Check sheet for the modelled part. Datum: model origin and axes. Units: mm. A direction names the side the tool comes from. Give positions to 0.01 mm unless a question says otherwise; leave off trailing zeros. Loops run counter-clockwise (first coordinate to the right, second up) from the corner with the lowest first, then second, coordinate; pieces in that order, holes last.
Autodesk Inventor part; units mm, degrees
ref_plane "YZ Plane" through (0, 0, 0) normal (1, 0, 0) x (0, 1, 0)
ref_plane "XZ Plane" through (0, 0, 0) normal (0, 1, 0) x (-1, 0, 0)
ref_plane "XY Plane" through (0, 0, 0) normal (0, 0, 1) x (1, 0, 0)
sketch "Sketch1" plane through (0, 0, 0) normal (0, 0, 1) x (1, 0, 0)
  line L0 (0, 0) -> (43.18, 0)
  line L1 (43.18, 0) -> (43.18, 22.86)
  line L2 (43.18, 22.86) -> (0, 22.86)
  line L3 (0, 22.86) -> (0, 0)
  dimension "d0" = 43.18
  dimension "d1" = 22.86
extrude "Extrusion1" add sketch "Sketch1" along normal blind 24.892
sketch "Sketch2" plane through (43.18, 0, 0) normal (1, 0, 0) x (0, 0, -1)
  line L0 (-4.826, 5.08) -> (-14.986, 5.08)
  line L1 (-14.986, 5.08) -> (-14.986, 17.78)
  line L2 (-14.986, 17.78) -> (-4.826, 17.78)
  line L3 (-4.826, 17.78) -> (-4.826, 5.08)
  line L4 (-24.892, 0) -> (-24.892, 22.86) construction
  line L5 (-14.986, 8.255) -> (-20.066, 8.255)
  line L6 (-20.066, 8.255) -> (-20.066, 14.605)
  line L7 (-20.066, 14.605) -> (-14.986, 14.605)
  line L8 (-14.986, 14.605) -> (-14.986, 8.255)
  line L9 (-20.066, 17.78) -> (-4.826, 17.78)
  line L10 (0, 22.86) -> (-24.892, 22.86) construction
  point P0 (0, 0)
  point P1 (-14.986, 11.43)
  point P2 (-24.892, 11.43)
  point P3 (-20.066, 11.43)
  point P4 (-12.446, 17.78)
  point P5 (-12.446, 22.86)
  dimension "d4" = 10.16
  dimension "d5" = 12.7
  dimension "d6" = 5.08
  dimension "d7" = 6.35
extrude "Extrusion2" cut sketch "Sketch2" against normal blind 12.7
sketch "Sketch3" plane through (0, 0, 0) normal (-1, 0, 0) x (0, 0, 1)
  line L0 (14.986, 14.605) -> (14.986, 17.78)
  line L1 (20.066, 14.605) -> (14.986, 14.605)
  line L2 (20.066, 8.255) -> (20.066, 14.605)
  line L3 (14.986, 8.255) -> (20.066, 8.255)
  line L4 (4.826, 5.08) -> (14.986, 5.08)
  line L5 (4.826, 17.78) -> (4.826, 5.08)
  line L6 (14.986, 17.78) -> (4.826, 17.78)
  line L7 (14.986, 5.08) -> (14.986, 8.255)
  point P0 (0, 0)
extrude "Extrusion3" cut sketch "Sketch3" against normal blind 12.7
properties part number "Ethernet Port" material "ABS Plastic"
(1) Section check A-A on z = 16.5. Record the boundary of the cut face in (x, y) (3 decimals).
(2) Section check B-B on x = 10.5. Record the boundary of the cut face in (y, z) (3 decimals).
(3) Material ranges on line 1 (Y direction, x = 7.5, z = 13); line 2 (Z direction, x = 37, y = 16.5); line 3 (X direction, y = 8.75, z = 7.75), recorded low to high.
(4) Release check for a two-part mould opening along Y. For faces 4 (the face through (22, 22.86, 12)), 5 (the face through (21, 0, 12)), 6 (the face through (6, 7, 14.986)) record: pulls with the +Y half, pulls with the -Y half, needs draft (parallel to the pull), parting line crosses it, or undercut.
(5) Gauge pin test, flat ends, axial feed: pin 1 Ø2 at (x, y) = (15.5, 11) entering from -Z; pin 2 Ø1.5 at (y, z) = (7.5, 10.5) entering from +X. Record the tip position at first contact, or that the pin passes through.
(6) Section check C-C on y = 16.5. Record the boundary of the cut face in (x, z), plus the area to 3 significant figures.
(7) Access from +Z, -Z, +X, -X, +Y, -Y to the whole of each face (thin tool, end or side, straight path). Record for faces 1 (the face through (6, 16, 14.986)), 2 (the face through (37, 16, 14.986)), 3 (the face through (21, 12, 24.892)).
Computed values:
1. outline: (0, 0) - (43.18, 0) - (43.18, 8.255) - (30.48, 8.255) - (30.48, 14.605) - (43.18, 14.605) - (43.18, 22.86) - (0, 22.86) - (0, 14.605) - (12.7, 14.605) - (12.7, 8.255) - (0, 8.255) - close
2. outline: (0, 0) - (22.86, 0) - (22.86, 24.892) - (0, 24.892) - close; hole (5.08, 4.826) - (17.78, 4.826) - (17.78, 14.986) - (14.605, 14.986) - (14.605, 20.066) - (8.255, 20.066) - (8.255, 14.986) - (5.08, 14.986) - close
3. line 1: y = 0 to 5.08, 17.78 to 22.86
3. line 2: z = 0 to 4.83, 14.99 to 24.89
3. line 3: x = 12.7 to 30.48
4. face 4: pulls with the +Y half
4. face 5: pulls with the -Y half
4. face 6: undercut
5. pin 1: stops at z = 0
5. pin 2: stops at x = 30.48
6. outline: (0, 0) - (43.18, 0) - (43.18, 4.83) - (30.48, 4.83) - (30.48, 14.99) - (43.18, 14.99) - (43.18, 24.89) - (0, 24.89) - (0, 14.99) - (12.7, 14.99) - (12.7, 4.83) - (0, 4.83) - close
6. area: 817 mm2
7. face 1: -X
7. face 2: +X
7. face 3: +Z, +X, -X, +Y, -Y
